Autodesk Inventor part; units mm, degrees
ref_plane "Plano de trabalho1" through (0, 0, 0) normal (0, -1, 0) x (1, 0, 0)
ref_plane "YZ Plane" through (0, 0, 0) normal (1, 0, 0) x (0, 1, 0)
ref_plane "XZ Plane" through (0, 0, 0) normal (0, 1, 0) x (-1, 0, 0)
sketch "Esboço1" plane through (0, 0, 0) normal (1, 0, 0) x (0, 1, 0)
  line L0 (0, 0) -> (10, 0)
  line L1 (10, 1) -> (1, 1)
  line L2 (10, 0) -> (10, -12)
  line L3 (10, -12) -> (1, -12)
  line L4 (10, 1) -> (11, 1)
  line L5 (11, 1) -> (11, -13)
  line L6 (11, -13) -> (1, -13)
  line L7 (0, 1) -> (0, 0)
  line L8 (10, 0) -> (0, 0)
  line L9 (1, -12) -> (0, -12)
  line L10 (0, -12) -> (0, -13)
  line L11 (1, -13) -> (0, -13)
  line L12 (1, 1) -> (0, 1)
extrude "Extrusão1" add sketch "Esboço1" along normal blind 20
ref_plane "Plano de trabalho1" through (0, 0, 0) normal (0, -1, 0) x (1, 0, 0)
sketch "Esboço2" plane through (0, 0, 0) normal (0, -1, 0) x (1, 0, 0)
  line L0 (0, 0) -> (20, 0)
  line L1 (20, 0) -> (20, -12)
  line L2 (20, -6) -> (22.0296, -6)
  line L3 (0, 1) -> (20, 1)
  line L4 (10, 1) -> (10, 5.0127) construction
  line L5 (7.6336, 1) -> (7.6336, 5.0127)
  line L6 (12.3664, 5.0127) -> (12.3664, 1)
  arc A0 (12.3664, 5.0127) -> (7.6336, 5.0127) centre (10, 5.0127) ccw
  circle A1 centre (10, 5.0127) radius 1.5
  line L7 (7.6336, -13) -> (7.6336, -17.0127)
  line L8 (12.3664, -17.0127) -> (12.3664, -13)
  arc A2 (7.6336, -17.0127) -> (12.3664, -17.0127) centre (10, -17.0127) ccw
  circle A3 centre (10, -17.0127) radius 1.5
  line L9 (12.3664, -13) -> (7.6336, -13)
  line L10 (0, -13) -> (20, -13)
  line L11 (12.3664, 1) -> (7.6336, 1)
  point P0 (10, 3.0064)
extrude "Extrusão2" add sketch "Esboço2" against normal blind 1
properties part number "engate_motor"
Model file for the job. Use its own axes, mm. A direction names the side the tool comes from. Coordinates: 2 decimals unless noted, no trailing zeros. Order: outer loops, then holes, each group sorted by start corner. A loop starts at its lowest first (then second) coordinate and runs counter-clockwise, first axis right, second up. Notation, with made-up numbers: M 59.5,-4.75 L 86.5,-4.75 A20 cw 86.5,9.25 Z; hole C -21,64 d8. An arc over 180 degrees is marked long. Answer as CSV lines item,"result".
(1) Band-saw the part on A-A, the plane y = 5.75. List the corners of the cut face in (x, z).
Geometry says:
outline,"M 0,-13 L 20,-13 L 20,-12 L 0,-12 Z; M 0,0 L 20,0 L 20,1 L 0,1 Z"
(2) Wall check: line 1 along Z through (x, y) = (10, 0.85); line 2 along Z through (x, y) = (11.75, 9); line 3 along Y through (x, z) = (12.25, -0.5). Give the ranges that are in metal, low to high.
Geometry says:
line 1,"z = -19.38 to -18.51, -15.51 to -12, 0 to 3.51, 6.51 to 7.38"
line 2,"z = -13 to -12, 0 to 1"
line 3,"y = 10 to 11"
(3) Flat gauge pins, fed straight in: pin 1 (4 mm diameter, centred on y = 5, z = -3.5, fed in from -X); pin 2 (1.1 mm diameter, centred on y = 0.5, z = -15.5, fed in from -X); pin 3 (1.5 mm diameter, centred on x = 2.5, z = -8.5, fed in from -Y); pin 4 (3.5 mm diameter, centred on x = 10, z = 5.01, fed in from +Y). Where does each tip first touch, or does it go through?
Geometry says:
pin 1,"passes through"
pin 2,"stops at x = 7.63"
pin 3,"stops at y = 10"
pin 4,"stops at y = 1"
(4) Band-saw the part on C-C, the plane z = 4.25. List the corners of the cut face in (x, y), then the cut area to 3 significant figures.
Geometry says:
outline,"M 7.63,0 L 8.71,0 L 8.71,1 L 7.63,1 Z; M 11.29,0 L 12.37,0 L 12.37,1 L 11.29,1 Z"
area,"2.15 mm2"
(5) Band-saw the part on B-B, the plane x = 10. List the corners of the cut face in (y, z), then the cut area to 3 significant figures.
Geometry says:
outline,"M 0,-19.38 L 1,-19.38 L 1,-18.51 L 0,-18.51 Z; M 0,-15.51 L 1,-15.51 L 1,-13 L 11,-13 L 11,1 L 1,1 L 1,3.51 L 0,3.51 L 0,0 L 10,0 L 10,-12 L 0,-12 Z; M 0,6.51 L 1,6.51 L 1,7.38 L 0,7.38 Z"
area,"40.8 mm2"
(6) Band-saw the part on D-D, the plane x = 13. List the corners of the cut face in (y, z).
Geometry says:
outline,"M 0,-13 L 11,-13 L 11,1 L 0,1 L 0,0 L 10,0 L 10,-12 L 0,-12 Z"
(7) Pull direction Z, two halves, no side cores. Call faces 1 (the flat face through (10, 10, -6)), 2 (the flat face through (20, 10.4, -7)), 3 (the cylindrical face through (10.05, 0.49, 7.38)), 4 (the cylindrical face through (8.81, 0.49, 4.1)): +Z half, -Z half, draft (parallel to the pull), parting line (faces both ways), or undercut.
Geometry says:
face 1,"undercut"
face 2,"draft"
face 3,"+Z half"
face 4,"undercut"
(8) 3-axis set-ups, long thin cutter, end or side, ignore diameter. For faces 5 (the flat face through (7.634, 0.5, -15)), 6 (the flat face through (12.366, 0.5, 3)), 7 (the flat face through (12.366, 0.5, -15)): which of +Z, -Z, +X, -X, +Y, -Y reach the whole face in a straight line?
Geometry says:
face 5,"-Z, -X, +Y, -Y"
face 6,"+Z, +X, +Y, -Y"
face 7,"-Z, +X, +Y, -Y"
